from build123d import *

# Parameters (mm, degrees)
SKETCH1_W           = 86
SKETCH1_H           = 86
SKETCH1_W_2         = 80
SKETCH1_H_2         = 80
BOSS_EXTRUDE1_DEPTH = 80
SKETCH2_W           = 86
SKETCH2_H           = 86
BOSS_EXTRUDE2_DEPTH = 3


with BuildPart() as part:
    # Sketch1 → Boss-Extrude1 (new body)
    with BuildSketch(Plane.XY):
        Rectangle(SKETCH1_W, SKETCH1_H)
        Rectangle(SKETCH1_W_2, SKETCH1_H_2, mode=Mode.SUBTRACT)
    extrude(amount=BOSS_EXTRUDE1_DEPTH)

    # Sketch2 → Boss-Extrude2 (add)
    with BuildSketch(Plane(origin=(0, 0, 0), x_dir=(-1, 0, 0), z_dir=(0, 0, -1))):
        Rectangle(SKETCH2_W, SKETCH2_H)
    extrude(amount=BOSS_EXTRUDE2_DEPTH)


solid = part.part
Build history of the part. All positions in model axes, mm. A direction names the side the tool comes from. Round coordinates to 2 decimals unless told otherwise and drop trailing zeros. Write each loop counter-clockwise with the first axis right and the second up, starting at its lowest first coordinate (ties: lowest second). Pieces come first, ordered by that corner, then holes. Notation, with made-up numbers: (1.25, -7) -> (20.25, -7) arc R29 ccw to (20.25, 14) -> close; hole circle Ø8 at (77.25, 21.5). An arc over 180 degrees is marked (long way). Use one line per item in the form item = value.
Q1. Drill centre lines: L1, parallel to X at y = -38, z = 14; L2, parallel to Z at x = 9.5, y = 6. Where is each one in solid material? Low to high.
Conclusion:
L1 = -43 to -40, 40 to 43
L2 = -3 to 0
Q2. Band-saw the part on A-A, the plane z = 4.5. Write the cut outline in (x, y).
Conclusion:
outline = (-43, -43) -> (43, -43) -> (43, 43) -> (-43, 43) -> close; hole (-40, -40) -> (40, -40) -> (40, 40) -> (-40, 40) -> close
Q3. Two-plate mould, pull along X, no slides. Class faces 1 (the flat face through (1, 43, 39)), 2 (the flat face through (-43, -1, 39)), 3 (the flat face through (-1, 40, 39)), 4 (the flat face through (40, -1, 39)): released by +X, released by -X, zero draft, split by the parting line, or undercut.
Conclusion:
face_1 = zero draft
face_2 = released by -X
face_3 = undercut
face_4 = undercut
Q4. Band-saw the part on B-B, the plane x = 2. Write the cut outline in (y, z).
Conclusion:
outline = (-43, -3) -> (43, -3) -> (43, 80) -> (40, 80) -> (40, 0) -> (-40, 0) -> (-40, 80) -> (-43, 80) -> close
Q5. Tool access for faces 5 (the flat face through (-40, -1, 39)), 6 (the flat face through (-3, -41, 80)): list every direction of +Z, -Z, +X, -X, +Y, -Y with a clear straight run to the whole face (end or side of a thin tool).
Conclusion:
face_5 = +Z
face_6 = +Z, +X, -X, +Y, -Y
Q6. Drop a flat-ended pin along its axis: P1, Ø8, axis at x = 4, y = 7, coming from the +Z side. Give the stop position or say it passes through.
Conclusion:
P1 = 0
